```python
from build123d import *

# Parameters (mm, degrees)
F0_W         = 139.7
F0_H         = 88.9
F1_DEPTH     = 76.2
F2_W         = 76.2
F2_H         = 38.1
F3_DEPTH     = 76.2
F4_W         = 114.3
F4_H         = 25.4
F5_DEPTH     = 76.2
F6_W         = 63.5
F6_H         = 50.8
F7_DEPTH     = 38.1
F8_R         = 31.74999
F9_R         = 38.09999
F10_T1_DEPTH = 25.4
F11_R        = 12.7
F12_DEPTH    = 25.4


# Not quite as in the source:
# - a fillet or chamfer that OpenCascade refuses, or shapes differently, is made with other operations: its cross-section is extruded or revolved along the edge and cut away or added
# - a fillet or chamfer is up to 0.001 mm smaller than in the source, because OpenCascade refuses the exact size


with BuildPart() as f1:
    # F0 (on Front) → F1 (new body)
    with BuildSketch(Plane.XZ):
        Rectangle(F0_W, F0_H)
    extrude(amount=F1_DEPTH)

    # F2 (on face) → F3 (cut)
    with BuildSketch(Plane.XZ.offset(76.2)):
        with Locations((31.75, 25.4)):
            Rectangle(F2_W, F2_H)
    extrude(amount=-F3_DEPTH, mode=Mode.SUBTRACT)

    # F4 (on face) → F5 (cut)
    with BuildSketch(Plane.XZ.offset(76.2)):
        with Locations((12.7, -31.75)):
            Rectangle(F4_W, F4_H)
    extrude(amount=-F5_DEPTH, mode=Mode.SUBTRACT)

    # F6 (on face) → F7 (cut)
    with BuildSketch(Plane.XY.offset(44.45)):
        with Locations((-38.1, -50.8)):
            Rectangle(F6_W, F6_H)
    extrude(amount=-F7_DEPTH, mode=Mode.SUBTRACT)

    # F8 (radius 31.75 in the source; OpenCascade refuses exactly that, so slightly less here)
    f8_edges = [f1.edges().sort_by_distance(p)[0] for p in [
        (-69.85, -12.7, 44.45),
        (-6.35, -12.7, 44.45),
    ]]
    fillet(f8_edges, radius=F8_R)

    # F9 (radius 38.1 in the source; OpenCascade refuses exactly that, so slightly less here)
    f9_edges = [f1.edges().sort_by_distance(p)[0] for p in [
        (69.85, -76.2, -6.35),
        (69.85, 0, -6.35),
    ]]
    fillet(f9_edges, radius=F9_R)

    # F10: fillet of radius 12.7 on 1 edges, made by hand

    # F10_s2 → F10_t1 (join)
    with BuildSketch(Plane.XZ):
        with BuildLine():
            ThreePointArc((5.894091852, 6.35), (-2.4200107012, 9.4497031955), (-6.6756486478, 17.2357167347))
            Line((-6.6756486478, 17.2357167347), (-7.9326226978, 17.0542884082))
            ThreePointArc((-7.9326226978, 17.0542884082), (-7.62, 12.70001), (-7.62, 6.35))
            Line((-7.62, 6.35), (-6.35, 5.08))
            Line((-6.35, 5.08), (5.894091852, 5.08))
            Line((5.894091852, 5.08), (5.894091852, 6.35))
        make_face()
    extrude(amount=F10_T1_DEPTH)

    # F11 (on face) → F12 (cut)
    with BuildSketch(Plane.XY.offset(6.35)):
        with Locations((31.75, -38.1)):
            Circle(F11_R)
    extrude(amount=-F12_DEPTH, mode=Mode.SUBTRACT)


solid = f1.part
```
CAD build for the part. Positions are in the model's coordinates, mm. A direction names the side the tool comes from. Coordinates: 2 decimals unless noted, no trailing zeros. Order: outer loops, then holes, each group sorted by start corner. A loop starts at its lowest first (then second) coordinate and runs counter-clockwise, first axis right, second up. Notation, with made-up numbers: M -30,-8.75 L 10,-8.75 A32 cw 10,25.25 Z; hole C 55,53 d8. An arc over 180 degrees is marked long. Answer as CSV lines item,"result".
1) Flat gauge pins, fed straight in: P1, Ø10, axis at x = 47.5, z = -14, coming from the -Y side; P2, Ø6, axis at x = -9, y = -67, coming from the +Z side; P3, Ø12.5, axis at y = -52, z = -36.5, coming from the +X side; P4, Ø5, axis at x = 0.5, z = 12, coming from the -Y side. Where does each tip first touch, or does it go through?
Verdict:
P1,"y = -74.65"
P2,"z = 6.35"
P3,"x = -44.45"
P4,"through"
2) Cut at C-C (x = -48.5). List the corners of the cut face in (y, z).
Verdict:
outline,"M -76.2,-44.45 L 0,-44.45 L 0,42.7 L -25.4,42.7 L -25.4,6.35 L -76.2,6.35 Z"
3) Drill centre lines: L1, parallel to Y at x = 31, z = -3; L2, parallel to Z at x = 49, y = -16; L3, parallel to X at y = -22, z = -26.5. Where is each one in solid material? Low to high. Write a range as from..to.
Verdict:
L1,"-76.2..-50.78, -25.42..0"
L2,"-19.05..6.35"
L3,"-69.85..-44.45"
4) Cut at B-B (y = -33). List the corners of the cut face in (x, z).
Verdict:
outline,"M -69.85,-44.45 L -44.45,-44.45 L -44.45,-19.05 L 20.12,-19.05 L 20.12,6.35 L -69.85,6.35 Z; M 43.38,-19.05 L 69.51,-19.05 L 69.51,6.35 L 43.38,6.35 Z"
5) Mould opens along Y. For faces 1 (the cylindrical face through (43.864, -34.285, -6.172)), 2 (the flat face through (-1, -46, 6.35)), 3 (the flat face through (-31, 0, 1)) say: released by +Y, released by -Y, zero draft, split by the parting line, or undercut.
Verdict:
face 1,"undercut"
face 2,"zero draft"
face 3,"released by +Y"
6) 3-axis set-ups, long thin cutter, end or side, ignore diameter. For faces 4 (the flat face through (-41, -25.4, 21)), 5 (the cylindrical face through (58.39, -10.86, -6.17)), 6 (the flat face through (12, -39, -19.05)): which of +Z, -Z, +X, -X, +Y, -Y reach the whole face in a straight line?
Verdict:
face 4,"+Z, +X, -X, -Y"
face 5,"+Z, -Z, +X, +Y"
face 6,"-Z, +X, +Y, -Y"
